from build123d import *

# Parameters (mm, degrees)
CUT_EXTRUDE1_REACH = 119.684
SKETCH2_R          = 1.975


with BuildPart() as part:
    # Sketch1 → Revolve1 (revolve)
    with BuildSketch(Plane(origin=(0, 0, 0), x_dir=(1, 0, 0), z_dir=(0, 1, 0)), mode=Mode.PRIVATE) as revolve1_sk:
        Polygon((0, 0), (23, 0), (23, 8.1), (13.2, 8.1), (13.2, 113.1), (10.2, 113.1), (10.2, 8.1), (0, 8.1), align=None)
    revolve(revolve1_sk.sketch.rotate(Axis((0, 0, -8.1), (0, 0, 1)), 180), axis=Axis((0, 0, -8.1), (0, 0, 1)))

    # Sketch2 → Cut-Extrude1 (cut, up to next)
    with BuildSketch(Plane.XY, mode=Mode.PRIVATE) as cut_extrude1_sk1:
        Circle(SKETCH2_R)
    cut_extrude1_tool1 = extrude(cut_extrude1_sk1.sketch, amount=-CUT_EXTRUDE1_REACH, mode=Mode.PRIVATE) & part.part
    add(cut_extrude1_tool1.solids().sort_by_distance((0, 0, 0))[0], mode=Mode.SUBTRACT)


solid = part.part
Can you work these out from the model? Positions are in its coordinate system, mm. A direction names the side the tool comes from. Give positions to 0.01 mm unless a question says otherwise; leave off trailing zeros. Loops run counter-clockwise (first coordinate to the right, second up) from the corner with the lowest first, then second, coordinate; pieces in that order, holes last. Notation, with made-up numbers: (50.5, 79) -> (80.5, 79) arc R23 ccw to (80.5, 114) -> close; hole circle Ø8 at (-28.75, 39). An arc over 180 degrees is marked (long way). Write item = value, one per line.
1) Suppose I cut it at C-C on x = 8.5. Write out the boundary of the cut face in (y, z), then the cut area to 3 significant figures.
Check result:
outline = (-21.37, -8.1) -> (-10.1, -8.1) -> (-10.1, -113.1) -> (-5.64, -113.1) -> (-5.64, -8.1) -> (5.64, -8.1) -> (5.64, -113.1) -> (10.1, -113.1) -> (10.1, -8.1) -> (21.37, -8.1) -> (21.37, 0) -> (-21.37, 0) -> close
area = 1,280 mm2
2) Will these pins go through, and if not, where does the flat tip stop? pin 1 (1.5 mm diameter, centred on x = 8.5, z = -17.5, fed in from -Y); pin 2 (1.5 mm diameter, centred on y = 15, z = -34.5, fed in from +X); pin 3 (8 mm diameter, centred on x = -6.5, z = -74, fed in from -Y); pin 4 (6 mm diameter, centred on x = 7.5, z = -98.5, fed in from -Y).
Check result:
pin_1 = -10.69
pin_2 = through
pin_3 = -12.96
pin_4 = -12.41
3) Suppose I cut it at A-A on y = 0. Write out the boundary of the cut face in (x, z) (3 decimals), then the cut area to 3 significant figures.
Check result:
outline = (-23, -8.1) -> (-13.2, -8.1) -> (-13.2, -113.1) -> (-10.2, -113.1) -> (-10.2, -8.1) -> (-1.975, -8.1) -> (-1.975, 0) -> (-23, 0) -> close; (1.975, -8.1) -> (10.2, -8.1) -> (10.2, -113.1) -> (13.2, -113.1) -> (13.2, -8.1) -> (23, -8.1) -> (23, 0) -> (1.975, 0) -> close
area = 971 mm2
4) Suppose I cut it at D-D on z = -87. Write out the boundary of the cut face in (x, y).
Check result:
outline = circle Ø26.4 at (0, 0); hole circle Ø20.4 at (0, 0)
5) I need wall thicknesses on L1, parallel to Y at x = 0, z = -4.75 (3 decimals); L2, parallel to Y at x = 0, z = -54; L3, parallel to Z at x = -4, y = -6. Which ranges of each line are inside material? Lowest first, please. Write a range as from..to.
Check result:
L1 = -23..-1.975, 1.975..23
L2 = -13.2..-10.2, 10.2..13.2
L3 = -8.1..0
6) Thinking about a two-plate mould opening in X: for faces 3 (the flat face through (-2.124, -0.143, -8.1)), 4 (the cylindrical face through (9.73, -8.92, -61.34)), 5 (the flat face through (5, 0, 0)), 6 (the cylindrical face through (-1.57, -1.2, -3.99)), which applies, released by +X, released by -X, zero draft, split by the parting line, or undercut?
Check result:
face_3 = undercut
face_4 = split by the parting line
face_5 = zero draft
face_6 = undercut
7) For faces 1 (the cylindrical face through (-9.73, -3.06, -59.86)), 2 (the cylindrical face through (2.994, -22.804, -4.107)), which set-ups out of +Z, -Z, +X, -X, +Y, -Y let a thin tool reach every point of the face, with its end or its side?
Check result:
face_1 = -Z
face_2 = +Z, -Z
